Source: three-view drawing plus pictorial views. Frame: mm from the lowest corner of the part. A direction names the side the tool comes from. Give positions to 0.01 mm unless a question says otherwise; leave off trailing zeros. Write each loop counter-clockwise with the first axis right and the second up, starting at its lowest first coordinate (ties: lowest second). Pieces come first, ordered by that corner, then holes.
Q1. Cut plane C-C on x = 67. Return the cut outline in (y, z), plus the area to 3 significant figures.
Q2. Draft query along X for the marked faces 4, 5, 6 and 7. Return one class per face: pulls with the +X half, pulls with the -X half, needs draft (parallel to the pull), parting line crosses it, or undercut.
Q3. Reachability of the marked faces 1, 2 and 3 from +Z, -Z, +X, -X, +Y, -Y: full face, straight path, thin tool, end or side. Return the list, or none.
Q4. Pin query (flat end, axial travel): pin 1 (12.5 mm diameter, centred on y = 34, z = 13, fed in from +X); pin 2 (6 mm diameter, centred on x = 20.5, z = 76, fed in from +Y); pin 3 (1 mm diameter, centred on y = 54.5, z = 27, fed in from +X); pin 4 (12 mm diameter, centred on x = 29.5, y = 69.5, fed in from -Z). Return the tip coordinate at first contact, or that it passes through.
Q5. Cut plane B-B on z = 28. Return the cut outline in (x, y) (1 decimal).
Q6. Line query: L1, parallel to Z at x = 34.5, y = 20; L2, parallel to X at y = 12.5, z = 9; L3, parallel to Y at x = 41, z = 10. Output: solid intervals per line, ascending.
Q7. Cut plane A-A on y = 61. Return the cut outline in (x, z), plus the area to 3 significant figures.
Q8. Cut plane D-D on z = 17.5. Return the cut outline in (x, y) (1 decimal), plus the area to 3 significant figures.
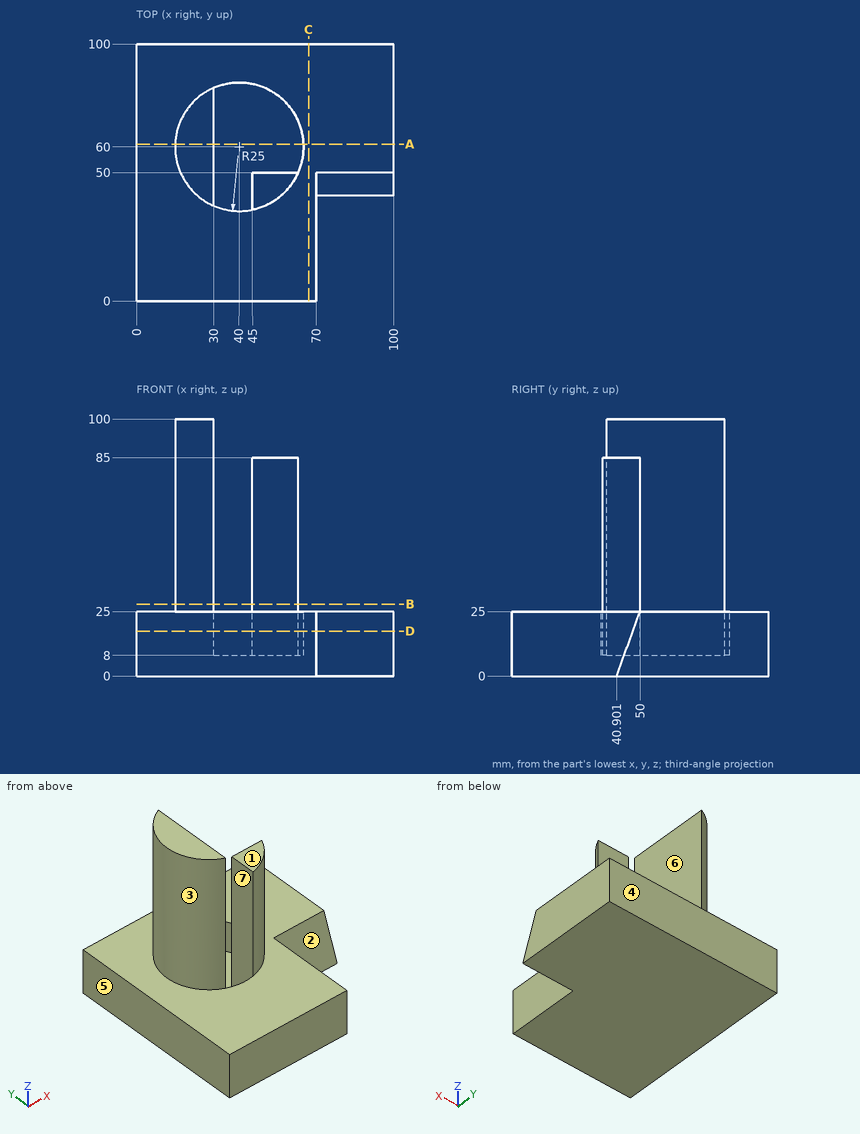
Data:
1. outline: (0, 0) - (100, 0) - (100, 25) - (0, 25) - close
1. area: 2,500 mm2
2. face 4: needs draft
2. face 5: pulls with the -X half
2. face 6: undercut
2. face 7: undercut
3. face 1: +Z, +X, +Y, -Y
3. face 2: +Z, +X, -Y
3. face 3: +Z, -X
4. pin 1: stops at x = 70
4. pin 2: stops at y = 78.78
4. pin 3: stops at x = 30
4. pin 4: stops at z = 0
5. outline: (30, 37.1) - (30, 82.9) arc R25 ccw to start; (45, 35.5) arc R25 ccw to (62.9, 50) - (45, 50) - close
6. L1: z = 0 to 25
6. L2: x = 0 to 70
6. L3: y = 0 to 35.02, 84.98 to 100
7. outline: (0, 0) - (100, 0) - (100, 25) - (64.98, 25) - (64.98, 8) - (30, 8) - (30, 100) - (15.02, 100) - (15.02, 25) - (0, 25) - close
7. area: 3,030 mm2
8. outline: (0, 0) - (70, 0) - (70, 47.3) - (100, 47.3) - (100, 100) - (0, 100) - close; hole (30, 37.1) arc R25 ccw to (45, 35.5) - (45, 50) - (62.9, 50) arc R25 ccw to (30, 82.9) - close
8. area: 7,290 mm2
